```python
from build123d import *

# Parameters (mm, degrees)
CROQUIS1_W                                  = 95
CROQUIS1_H                                  = 40
SALIENTE_EXTRUIR1_DEPTH                     = 5
SALIENTE_EXTRUIR2_DEPTH                     = 40
CROQUIS3_W                                  = 95
CROQUIS3_H                                  = 2
SALIENTE_EXTRUIR3_DEPTH                     = 2
CROQUIS4_W                                  = 95
CROQUIS4_H                                  = 2
SALIENTE_EXTRUIR4_DEPTH                     = 2
DI_METRO_DE_TALADRO_2_0_2_1_D               = 2
DI_METRO_DE_TALADRO_2_0_2_1_DEPTH           = 10
DI_METRO_DE_TALADRO_2_0_2_1_TIP             = 0.600860619
DI_METRO_DE_TALADRO_2_0_2_2_D               = 2
DI_METRO_DE_TALADRO_2_0_2_2_DEPTH           = 10
DI_METRO_DE_TALADRO_2_0_2_2_TIP             = 0.600860619
DI_METRO_DE_TALADRO_2_0_2_2_ON_FACE_2_D     = 2
DI_METRO_DE_TALADRO_2_0_2_2_ON_FACE_2_DEPTH = 10
DI_METRO_DE_TALADRO_2_0_2_2_ON_FACE_2_TIP   = 0.600860619


with BuildPart() as part:
    # Croquis1 → Saliente-Extruir1 (new body)
    with BuildSketch(Plane(origin=(0, 0, 0), x_dir=(1, 0, 0), z_dir=(0, 1, 0))):
        with Locations((47.5, 20)):
            Rectangle(CROQUIS1_W, CROQUIS1_H)
    extrude(amount=SALIENTE_EXTRUIR1_DEPTH)

    # Croquis2 → Saliente-Extruir2 (add)
    with BuildSketch(Plane(origin=(0, 5, 0), x_dir=(1, 0, 0), z_dir=(0, 1, 0))):
        Polygon((0, 35), (90, 35), (90, 0), (95, 0), (95, 40), (0, 40), align=None)
    extrude(amount=SALIENTE_EXTRUIR2_DEPTH)

    # Croquis3 → Saliente-Extruir3 (add)
    with BuildSketch(Plane(origin=(0, 45, 0), x_dir=(1, 0, 0), z_dir=(0, 1, 0))):
        with Locations((47.5, 37.5)):
            Rectangle(CROQUIS3_W, CROQUIS3_H)
    extrude(amount=SALIENTE_EXTRUIR3_DEPTH)

    # Croquis4 → Saliente-Extruir4 (add)
    with BuildSketch(Plane.XY):
        with Locations((47.5, 2.5)):
            Rectangle(CROQUIS4_W, CROQUIS4_H)
    extrude(amount=SALIENTE_EXTRUIR4_DEPTH)

    # Diámetro de taladro Ø2.0 (2)1
    with Locations(Plane(origin=(0, 42.5, -37.5), x_dir=(0, 0, -1), z_dir=(-1, 0, 0))):
        with Locations((0, 0), (-35, 40)):
            Hole(DI_METRO_DE_TALADRO_2_0_2_1_D / 2, depth=DI_METRO_DE_TALADRO_2_0_2_1_DEPTH)
            with Locations((0, 0, -(DI_METRO_DE_TALADRO_2_0_2_1_DEPTH + DI_METRO_DE_TALADRO_2_0_2_1_TIP / 2))):  # 118° drill point
                Cone(0, DI_METRO_DE_TALADRO_2_0_2_1_D / 2, DI_METRO_DE_TALADRO_2_0_2_1_TIP, mode=Mode.SUBTRACT)

    # Diámetro de taladro Ø2.0 (2)2
    with Locations(Plane(origin=(92.5, 45, -32.5), x_dir=(0, 0, 1), z_dir=(0, 1, 0))):
        with Locations((0, 0)):
            Hole(DI_METRO_DE_TALADRO_2_0_2_2_D / 2, depth=DI_METRO_DE_TALADRO_2_0_2_2_DEPTH)
            with Locations((0, 0, -(DI_METRO_DE_TALADRO_2_0_2_2_DEPTH + DI_METRO_DE_TALADRO_2_0_2_2_TIP / 2))):  # 118° drill point
                Cone(0, DI_METRO_DE_TALADRO_2_0_2_2_D / 2, DI_METRO_DE_TALADRO_2_0_2_2_TIP, mode=Mode.SUBTRACT)

    # Diámetro de taladro Ø2.0 (2)2 on face 2
    with Locations(Plane(origin=(92.5, 7.5, 0), x_dir=(1, 0, 0), z_dir=(0, 0, 1))):
        with Locations((0, 0)):
            Hole(DI_METRO_DE_TALADRO_2_0_2_2_ON_FACE_2_D / 2, depth=DI_METRO_DE_TALADRO_2_0_2_2_ON_FACE_2_DEPTH)
            with Locations((0, 0, -(DI_METRO_DE_TALADRO_2_0_2_2_ON_FACE_2_DEPTH + DI_METRO_DE_TALADRO_2_0_2_2_ON_FACE_2_TIP / 2))):  # 118° drill point
                Cone(0, DI_METRO_DE_TALADRO_2_0_2_2_ON_FACE_2_D / 2, DI_METRO_DE_TALADRO_2_0_2_2_ON_FACE_2_TIP, mode=Mode.SUBTRACT)


solid = part.part
```
The model under review builds one solid part; all positions refer to its coordinate system, in mm. A direction names the side the tool comes from. Give positions to 0.01 mm unless a question says otherwise; leave off trailing zeros. Order: outer loops, then holes, each group sorted by start corner. A loop starts at its lowest first (then second) coordinate and runs counter-clockwise, first axis right, second up. Notation, with made-up numbers: (13, -27.5) - (60, -27.5) arc R14 cw to (60, -2.5) - close; hole circle Ø6 at (-15.5, 8.5). An arc over 180 degrees is marked (long way). Use CSV: the item, a comma, the result in double quotes. Start each with the question number.
Q1. To check wall thickness, follow line 1 along Y through (x, z) = (5.5, -2.5); line 2 along X through (y, z) = (7.5, -2.5); line 3 along Y through (x, z) = (2.5, -37.5). State the ranges of each line that lie inside material, in increasing order. Write a range as [from, to].
Q2. We need section C-C, the plane z = -14.5. Write out the cut boundary in (x, y).
Q3. Clearance check with flat-ended pins moving along their axes: pin 1 Ø21 at (x, y) = (44, 30.5) entering from +Z; pin 2 Ø11 at (x, z) = (37.5, -9.5) entering from +Y; pin 3 Ø3 at (y, z) = (17.5, -19.5) entering from -X. State where each tip first meets the part, or that it passes through.
Q4. The part is to be moulded in two halves that separate along X. For faces 5 (the flat face through (95, 23, -19)), 6 (the flat face through (47, 1.5, 1)), 7 (the cylindrical face through (93.5, 7.5, -5.1)), say which applies: +X half, -X half, draft (parallel to the pull), parting line (faces both ways), or undercut.
Q5. We need section B-B, the plane x = 45. Write out the cut boundary in (y, z).
Q6. We need section D-D, the plane y = 17. Write out the cut boundary in (x, z), and give its area (3 significant figures).
Q7. We need section A-A, the plane z = -8.5. Write out the cut boundary in (x, y), and give its area (3 significant figures).
Q8. Tool access review of faces 1 (the flat face through (47, 46, -36.5)), 2 (the flat face through (47, 46, -38.5)), 3 (the cylindrical face through (5.1, 3.1, -3.3)), 4 (the flat face through (44, 5, -18)): name each direction out of +Z, -Z, +X, -X, +Y, -Y from which nothing blocks a thin tool from reaching the whole face with its end or side.
Outcome:
1,line 1,"y = [0, 1.5], [3.5, 5]"
1,line 2,"x = [90, 91.5], [93.5, 95]"
1,line 3,"y = [0, 41.5], [43.5, 47]"
2,outline,"(0, 0) - (95, 0) - (95, 45) - (90, 45) - (90, 5) - (0, 5) - close"
3,pin 1,"stops at z = -35"
3,pin 2,"stops at y = 5"
3,pin 3,"stops at x = 90"
4,face 5,"+X half"
4,face 6,"draft"
4,face 7,"undercut"
5,outline,"(0, -40) - (45, -40) - (45, -38.5) - (47, -38.5) - (47, -36.5) - (45, -36.5) - (45, -35) - (5, -35) - (5, 0) - (3.5, 0) - (3.5, 2) - (1.5, 2) - (1.5, 0) - (0, 0) - close"
6,outline,"(0, -40) - (95, -40) - (95, 0) - (90, 0) - (90, -35) - (0, -35) - close"
6,area,"650 mm^2"
7,outline,"(0, 0) - (95, 0) - (95, 45) - (90, 45) - (90, 5) - (0, 5) - close; hole circle Ø2 at (92.5, 7.5)"
7,area,"672 mm^2"
8,face 1,"+Z, +X, -X, +Y"
8,face 2,"-Z, +X, -X, +Y"
8,face 3,"-X"
8,face 4,"+Z, -X, +Y"
